Design review of the part built by this model. Coordinates are the model's own, in mm. A direction names the side the tool comes from. Round coordinates to 2 decimals unless told otherwise and drop trailing zeros. Order: outer loops, then holes, each group sorted by start corner. A loop starts at its lowest first (then second) coordinate and runs counter-clockwise, first axis right, second up. Notation, with made-up numbers: (-37.5, 2) - (-29.5, 2) arc R4 ccw to (-29.5, 9) - close; hole circle Ø8 at (78, -18). An arc over 180 degrees is marked (long way). Write item = value, one per line.
from build123d import *

# Parameters (mm, degrees)
SKETCH1_W                    = 15
SKETCH1_H                    = 30
SKETCH1_R                    = 2.1
BASE_FLANGE1_DEPTH           = 0.5
EDGE_FLANGE1_STRIP_W         = 3.4732
EDGE_FLANGE1_STRIP_H         = 0.5
EDGE_FLANGE1_STRIP_CUT_DEPTH = 30
EDGE_FLANGE1_DEPTH           = 30
SKETCH8_R                    = 1.1
CUT_EXTRUDE1_DEPTH           = 10


# Sheet-metal steps are written as plain solids
with BuildPart() as part:
    # Sketch1 → Base-Flange1 (new body)
    with BuildSketch(Plane(origin=(0, 0, 0), x_dir=(1, 0, 0), z_dir=(0, 1, 0))):
        with Locations((10.481024164, 1.814426404)):
            Rectangle(SKETCH1_W, SKETCH1_H)
        with Locations(Location((13.058795971, -5.685573596, 0), (0, 0, 270))):
            Circle(SKETCH1_R, mode=Mode.SUBTRACT)
        with Locations(Location((13.058795971, 9.314426404, 0), (0, 0, 270))):
            Circle(SKETCH1_R, mode=Mode.SUBTRACT)
    extrude(amount=-BASE_FLANGE1_DEPTH)

    # Edge-Flange1 strip (across the edge) → Edge-Flange1 strip cut (cut)
    with BuildSketch(Plane(origin=(2.981024164, -0.5, 13.185573596), x_dir=(1, 0, 0), z_dir=(0, 0, -1))):
        with Locations((-1, -0.25)):
            Rectangle(EDGE_FLANGE1_STRIP_W, EDGE_FLANGE1_STRIP_H)
    extrude(amount=EDGE_FLANGE1_STRIP_CUT_DEPTH, mode=Mode.SUBTRACT)

    # Edge-Flange1 section (across the edge) → Edge-Flange1 (add)
    with BuildSketch(Plane(origin=(2.981024164, -0.5, 13.185573596), x_dir=(1, 0, 0), z_dir=(0, 0, -1))):
        with BuildLine():
            Line((-0.5, 0.7366), (-0.5, 5))
            Line((-0.5, 5), (0, 5))
            Line((0, 5), (0, 0.7366))
            ThreePointArc((0, 0.7366), (0.215745145, 0.215745145), (0.7366, 0))
            Line((0.7366, 0), (0.7366, -0.5))
            ThreePointArc((0.7366, -0.5), (-0.137808246, -0.137808246), (-0.5, 0.7366))
        make_face()
    extrude(amount=EDGE_FLANGE1_DEPTH)

    # Sketch8 → Cut-Extrude1 (cut)
    with BuildSketch(Plane(origin=(2.981024164, 0, 0), x_dir=(0, 0, -1), z_dir=(1, 0, 0))):
        with Locations(Location((5.114426404, -3.5, 0), (0, 0, 90))):
            Circle(SKETCH8_R)
        with Locations(Location((-1.485573596, -3.5, 0), (0, 0, 90))):
            Circle(SKETCH8_R)
    extrude(amount=-CUT_EXTRUDE1_DEPTH, mode=Mode.SUBTRACT)


solid = part.part
1) We need section B-B on z = -9. Write out the cut boundary in (x, y), and give its area (3 significant figures).
Findings:
outline = (2.48, -5.5) - (2.98, -5.5) - (2.98, -1.24) arc R0.74 cw to (3.72, -0.5) - (10.98, -0.5) - (10.98, 0) - (3.72, 0) arc R1.24 ccw to (2.48, -1.24) - close; (15.14, -0.5) - (17.98, -0.5) - (17.98, 0) - (15.14, 0) - close
area = 7.96 mm^2
2) We need section D-D on x = 5.25. Write out the cut boundary in (y, z), and give its area (3 significant figures).
Findings:
outline = (-0.5, -16.81) - (0, -16.81) - (0, 13.19) - (-0.5, 13.19) - close
area = 15.0 mm^2
3) We need section C-C on z = 10.75. Write out the cut boundary in (x, y).
Findings:
outline = (2.48, -5.5) - (2.98, -5.5) - (2.98, -1.24) arc R0.74 cw to (3.72, -0.5) - (17.98, -0.5) - (17.98, 0) - (3.72, 0) arc R1.24 ccw to (2.48, -1.24) - close
4) We need section A-A on y = -3.5. Write out the cut boundary in (x, z).
Findings:
outline = (2.48, -16.81) - (2.98, -16.81) - (2.98, -6.21) - (2.48, -6.21) - close; (2.48, -4.01) - (2.98, -4.01) - (2.98, 0.39) - (2.48, 0.39) - close; (2.48, 2.59) - (2.98, 2.59) - (2.98, 13.19) - (2.48, 13.19) - close
5) The part is to be moulded in two halves that separate along Z. For faces 3 (the flat face through (11, 0, -2)), 4 (the flat face through (8, -0.3, -16.814)), 5 (the cylindrical face through (11.01, -0.25, 5.23)), say which applies: released by +Z, released by -Z, zero draft, split by the parting line, or undercut.
Findings:
face_3 = zero draft
face_4 = released by -Z
face_5 = undercut
6) Clearance check with flat-ended pins moving along their axes: pin 1 Ø3 at (y, z) = (-3.5, 1.49) entering from +X; pin 2 Ø4.5 at (x, z) = (10, -3) entering from -Y. State where each tip first meets the part, or that it passes through.
Findings:
pin_1 = 2.98
pin_2 = -0.5
7) For faces 1 (the flat face through (11, -0.5, -2)), 2 (the flat face through (8, -0.3, 13.186)), list the 3-axis set-ups (+Z, -Z, +X, -X, +Y, -Y) from which the entire face can be reached by the end or side of a thin tool; tool diameter is ignored.
Findings:
face_1 = +Z, -Z, +X, -Y
face_2 = +Z, +X, -X, +Y, -Y
8) To check wall thickness, follow L1, parallel to Z at x = 2.9, y = -3.5; L2, parallel to Y at x = 7.5, z = -10.25; L3, parallel to X at y = -4.4, z = -9.5. State the ranges of each line that lie inside material, in increasing order. Write a range as from..to.
Findings:
L1 = -16.81..-6.21, -4.01..0.39, 2.59..13.19
L2 = -0.5..0
L3 = 2.48..2.98
